from build123d import *

# Parameters (mm, degrees)
SKIZZE1_W                       = 155
SKIZZE1_H                       = 48
AUFSATZ_LINEAR_AUSTRAGEN1_DEPTH = 28
VERRUNDUNG1_R                   = 5


with BuildPart() as part:
    # Skizze1 → Aufsatz-Linear austragen1 (new body)
    with BuildSketch(Plane(origin=(0, 0, 0), x_dir=(1, 0, 0), z_dir=(0, 1, 0))):
        with Locations((77.5, 24)):
            Rectangle(SKIZZE1_W, SKIZZE1_H)
    extrude(amount=AUFSATZ_LINEAR_AUSTRAGEN1_DEPTH)

    # Verrundung1
    verrundung1_edges = [part.edges().sort_by_distance(p)[0] for p in [
        (155, 28, -24),
        (77.5, 28, -48),
        (0, 28, -24),
        (77.5, 0, -48),
        (155, 0, -24),
        (77.5, 0, 0),
        (0, 0, -24),
        (0, 14, -48),
        (155, 14, -48),
        (155, 14, 0),
        (0, 14, 0),
        (77.5, 28, 0),
    ]]
    fillet(verrundung1_edges, radius=VERRUNDUNG1_R)


solid = part.part
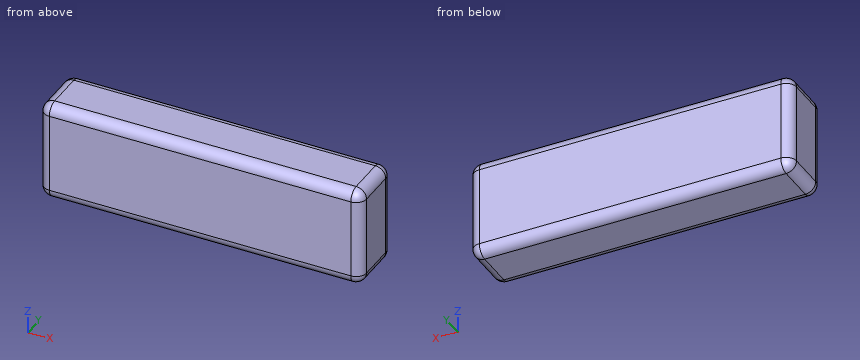
The listing builds one solid part. Answer for the finished solid, in the listing's coordinates (mm). Coordinates: 2 decimals unless noted, no trailing zeros. Write each loop counter-clockwise with the first axis right and the second up, starting at its lowest first coordinate (ties: lowest second). Pieces come first, ordered by that corner, then holes. Notation, with made-up numbers: (49, 16.5) - (90, 16.5) arc R26 cw to (90, 42.5) - close; hole circle Ø6 at (-2.5, -37.5). An arc over 180 degrees is marked (long way). Answer as CSV lines item,"result".
1. Find section A-A (x = 81.5). Give the vertices of the cut face in (y, z).
Computed values:
outline,"(0, -43) arc R5 ccw to (5, -48) - (23, -48) arc R5 ccw to (28, -43) - (28, -5) arc R5 ccw to (23, 0) - (5, 0) arc R5 ccw to (0, -5) - close"
2. Straight lines are drawn through the part: line 1 (Z direction, x = 131, y = 23.5); line 2 (Y direction, x = 88, z = -43.5); line 3 (X direction, y = 25.5, z = -20). For each, find the intervals that lie inside material, in ascending order. Write a range as [from, to].
Computed values:
line 1,"z = [-47.97, -0.03]"
line 2,"y = [0.03, 27.97]"
line 3,"x = [0.67, 154.33]"
3. Given P1, Ø1.5, axis at x = 88.5, y = 4, coming from the -Z side, flat-ended and moving along its own axis, determine where the tip first touches the part or whether it passes through.
Computed values:
P1,"stops at z = -47.99"
4. Find section B-B (z = -3.5). Give the vertices of the cut face in (x, y).
Computed values:
outline,"(0.23, 5) arc R4.77 ccw to (5, 0.23) - (150, 0.23) arc R4.77 ccw to (154.77, 5) - (154.77, 23) arc R4.77 ccw to (150, 27.77) - (5, 27.77) arc R4.77 ccw to (0.23, 23) - close"
